Can you work these out from the model? Positions are in its coordinate system, mm. A direction names the side the tool comes from. Give positions to 0.01 mm unless a question says otherwise; leave off trailing zeros. Order: outer loops, then holes, each group sorted by start corner. A loop starts at its lowest first (then second) coordinate and runs counter-clockwise, first axis right, second up.
Item 1: Which directions (+Z, -Z, +X, -X, +Y, -Y) give clear straight access to the entire face, cutting with the end or side of a thin tool? Please do faces 5 (the flat face through (2, -2, 6)), 6 (the flat face through (4.3, -2.1, 3)).
Item 2: I want a section at A-A, the plane x = 0. Write out the boundary of the cut face in (y, z), then the cut area to 3 significant figures.
Item 3: I want a section at D-D, the plane y = 4.25. Write out the boundary of the cut face in (x, z).
Item 4: If I drill on line 1 along Y through (x, z) = (-1.5, 2.75); line 2 along Y through (x, z) = (0, 3.65); line 3 along Y through (x, z) = (0, 2.9), over which ranges is the centre line in solid material (lowest first)?
Item 5: I'm going to push flat-ended pins straight in: pin 1 Ø10 at (x, y) = (3, -5) entering from -Z; pin 2 Ø1 at (x, z) = (-2.5, 4) entering from -Y; pin 3 Ø5 at (x, y) = (-3, 8) entering from +Z. Where does each tip first touch, or does it pass through?
Item 6: I want a section at C-C, the plane z = 0.6. Write out the boundary of the cut face in (x, y).
Item 7: If we mould it in two halves opening along X, with no side actions, what happens to faces 1 (the cylindrical face through (-0.59, 4.46, 4.48)), 2 (the cylindrical face through (0.54, -2.44, 2.96)), 3 (the flat face through (2, -2, 0)), 4 (the cylindrical face through (-1.306, -5.409, 1.521))? For each: +X half, -X half, draft (parallel to the pull), parting line (faces both ways), or undercut.
```python
from build123d import *

# Parameters (mm, degrees)
SKETCH1_R             = 10
BOSS_EXTRUDE1_DEPTH   = 3
SKETCH2_R             = 4.5
BOSS_EXTRUDE2_DEPTH   = 3
F_3_0MM_DOWEL_HOLE1_D = 3
F_5_0MM_DOWEL_HOLE1_D = 5


with BuildPart() as part:
    # Sketch1 → Boss-Extrude1 (new body)
    with BuildSketch(Plane.XY):
        Circle(SKETCH1_R)
    extrude(amount=BOSS_EXTRUDE1_DEPTH)

    # Sketch2 → Boss-Extrude2 (add)
    with BuildSketch(Plane.XY.offset(3)):
        Circle(SKETCH2_R)
    extrude(amount=BOSS_EXTRUDE2_DEPTH)

    # Ø3.0mm Dowel Hole1 (through all)
    with Locations(Plane(origin=(0, 0, 0), x_dir=(-1, 0, 0), z_dir=(0, 0, -1))):
        with Locations((6.673703276, 2.112270007), (2.112270007, -6.673703276), (-6.673703276, -2.112270007), (-2.112270007, 6.673703276)):
            Hole(F_3_0MM_DOWEL_HOLE1_D / 2)

    # Ø5.0mm Dowel Hole1 (through all)
    with Locations(Plane.XY.offset(6)):
        with Locations((0, 0)):
            Hole(F_5_0MM_DOWEL_HOLE1_D / 2)


solid = part.part
```
Results list:
1. face 5: +Z, +X, -X, +Y, -Y
1. face 6: +Z
2. outline: (-10, 0) - (-2.5, 0) - (-2.5, 6) - (-4.5, 6) - (-4.5, 3) - (-10, 3) - close; (2.5, 0) - (10, 0) - (10, 3) - (4.5, 3) - (4.5, 6) - (2.5, 6) - close
2. area: 57.0 mm2
3. outline: (-9.05, 0) - (9.05, 0) - (9.05, 3) - (1.48, 3) - (1.48, 6) - (-1.48, 6) - (-1.48, 3) - (-9.05, 3) - close
4. line 1: y = -9.89 to -8.04, -5.3 to -2, 2 to 9.89
4. line 2: y = -4.5 to -2.5, 2.5 to 4.5
4. line 3: y = -10 to -2.5, 2.5 to 10
5. pin 1: stops at z = 0
5. pin 2: stops at y = -4.03
5. pin 3: stops at z = 3
6. outline: circle Ø20 at (0, 0); hole circle Ø3 at (-6.67, 2.11); hole circle Ø3 at (-2.11, -6.67); hole circle Ø5 at (0, 0); hole circle Ø3 at (2.11, 6.67); hole circle Ø3 at (6.67, -2.11)
7. face 1: parting line
7. face 2: undercut
7. face 3: draft
7. face 4: undercut
